Design review of the part built by this model. Coordinates are the model's own, in mm. A direction names the side the tool comes from. Round coordinates to 2 decimals unless told otherwise and drop trailing zeros. Loops run counter-clockwise (first coordinate to the right, second up) from the corner with the lowest first, then second, coordinate; pieces in that order, holes last. Notation, with made-up numbers: (48, 20) - (92, 20) arc R30 ccw to (92, 47) - close; hole circle Ø11 at (39, 54). An arc over 180 degrees is marked (long way). One line per question, with ' | ' between items. Start each with the question number.
Autodesk Inventor part; units mm, degrees
ref_plane "YZ Plane" through (0, 0, 0) normal (1, 0, 0) x (0, 1, 0)
ref_plane "XZ Plane" through (0, 0, 0) normal (0, 1, 0) x (-1, 0, 0)
ref_plane "XY Plane" through (0, 0, 0) normal (0, 0, 1) x (1, 0, 0)
sketch "Sketch1" plane through (0, 0, 0) normal (0, 0, 1) x (1, 0, 0)
  line L0 (-12.1708, 16.0073) -> (13.2292, 16.0073)
  line L1 (13.2292, 16.0073) -> (13.2292, -34.7927)
  line L2 (13.2292, -34.7927) -> (-12.1708, -34.7927)
  line L3 (-12.1708, -34.7927) -> (-12.1708, 16.0073)
  line L4 (11.9592, 14.7373) -> (-10.9008, 14.7373)
  line L5 (-10.9008, 14.7373) -> (-10.9008, -33.5227)
  line L6 (-10.9008, -33.5227) -> (11.9592, -33.5227)
  line L7 (11.9592, -33.5227) -> (11.9592, 14.7373)
  point P0 (0, 0)
  dimension "d0" = 25.4
  dimension "d1" = 50.8
  dimension "d2" = 1.27
extrude "Extrusion1" add sketch "Sketch1" along normal blind 292.1
sketch "Sketch2" plane through (-12.1708, 16.0073, 0) normal (0, 1, 0) x (1, 0, 0)
  circle A0 centre (12.7, -12.7) radius 1.7272
  line L0 (25.4, 0) -> (0, 0)
  line L1 (0, 0) -> (0, -292.1)
  point P0 (12.1708, 0)
  dimension "d5" = 3.4544
  dimension "d6" = 12.7
  dimension "d7" = 12.7
extrude "Extrusion2" cut sketch "Sketch2" against normal through all
pattern_linear "Rectangular Pattern1" count 12 spacing 25.4 along (0, 0, 1) of "Extrusion2"
sketch "Sketch4" plane through (13.2292, -34.7927, 0) normal (1, 0, 0) x (0, 0, -1)
  circle A0 centre (-266.7, 25.4) radius 14.2875
  line L0 (0, 0) -> (0, 50.8)
  line L1 (0, 50.8) -> (-292.1, 50.8)
  point P0 (0, 34.7927)
  dimension "d21" = 266.7
  dimension "d22" = 25.4
  dimension "d23" = 28.575
extrude "Extrusion4" cut sketch "Sketch4" against normal through all
sketch "Sketch5" plane through (13.2292, -34.7927, 0) normal (1, 0, 0) x (0, 0, -1)
  circle A0 centre (-165.1, 25.4) radius 25.4 construction
  circle A1 centre (-165.1, 25.4) radius 9.525
  circle A2 centre (-190.5, 25.4) radius 2.5781
  circle A3 centre (-139.7, 25.4) radius 2.5781
  line L0 (0, 0) -> (0, 50.8)
  line L1 (0, 50.8) -> (-292.1, 50.8)
  line L2 (-190.5, 25.4) -> (-139.7, 25.4) construction
  point P0 (0, 34.7927)
  dimension "d26" = 165.1
  dimension "d27" = 19.05
  dimension "d28" = 25.4
  dimension "d29" = 50.8
  dimension "d30" = 5.1562
extrude "Extrusion5" cut sketch "Sketch5" against normal through all
equation "\"d3\" = d13"
equation "\"d10\" = d14"
equation "\"d31\" = d27"
equation "\"d13\" = 292.1"
equation "\"d14\" = 11.5"
properties part number "VerseFrame 10.5in Uptake support"
1. The part is to be moulded in two halves that separate along Z. For faces 3 (the face through (1, 14.737, 144)), 4 (the face through (12.603, -9.279, 193.076)), 5 (the face through (12.2, -9.3, 292.1)), say which applies: pulls with the +Z half, pulls with the -Z half, needs draft (parallel to the pull), parting line crosses it, or undercut.
2. Take a section at A-A, the plane x = -8.5. Give the boundary of the cut face in (y, z).
3. To check wall thickness, follow line 1 along X through (y, z) = (15.15, 12.7); line 2 along X through (y, z) = (-18, 231); line 3 along Y through (x, z) = (11, 109.5). State the ranges of each line that lie inside material, in increasing order.
4. Machinability: for faces 1 (the face through (11.959, -10, 144)), 2 (the face through (-11.527, -9.279, 193.076)), which of the approach directions +Z, -Z, +X, -X, +Y, -Y give a long, thin tool a straight path to every point of the face, cutting with its end or side? Answer none if there is none.
5. Clearance check with a flat-ended pin moving along its axis: P1, Ø3, axis at x = 0.53, z = 241.3, coming from the +Y side. State where the tip first meets the part, or that it passes through.
6. Take a section at B-B, the plane y = -31. Give the boundary of the cut face in (x, z).
Answer list:
1) face 3: needs draft | face 4: undercut | face 5: pulls with the +Z half
2) outline: (-34.79, 0) - (-33.52, 0) - (-33.52, 292.1) - (-34.79, 292.1) - close; (14.74, 0) - (16.01, 0) - (16.01, 292.1) - (14.74, 292.1) - close
3) line 1: x = -12.17 to -1.2, 2.26 to 13.23 | line 2: x = -12.17 to -10.9, 11.96 to 13.23 | line 3: y = -34.79 to -33.52, 14.74 to 16.01
4) face 1: +Z, -Z | face 2: +X, -X
5) P1: passes through
6) outline: (-12.17, 0) - (-10.9, 0) - (-10.9, 292.1) - (-12.17, 292.1) - close; (11.96, 0) - (13.23, 0) - (13.23, 292.1) - (11.96, 292.1) - close
